Geometry check sheet. Reference: the model listing, model coordinates, mm. A direction names the side the tool comes from. Give positions to 0.01 mm unless a question says otherwise; leave off trailing zeros. Order: outer loops, then holes, each group sorted by start corner. A loop starts at its lowest first (then second) coordinate and runs counter-clockwise, first axis right, second up. Notation, with made-up numbers: M 55,17.25 L 68,17.25 A27 ccw 68,36.25 Z; hole C -36,-24.75 d5. An arc over 180 degrees is marked long. Answer as CSV lines item,"result". Start each with the question number.
Q1. Go/stop test with flat-tipped pins: pin 1 (6.5 mm diameter, centred on x = 4.5, y = 51.5, fed in from -Z); pin 2 (6 mm diameter, centred on x = -1.5, z = 31.5, fed in from +Y); pin 3 (5 mm diameter, centred on x = -20, z = 32, fed in from -Y). Record where each tip stops, or that it passes through.
Q2. Section check D-D, the plane y = 57. Record the boundary of the cut face in (x, z).
Q3. Section check A-A, the plane y = 43. Record the boundary of the cut face in (x, z) (3 decimals).
Q4. Thickness scan on line 1 (Y direction, x = -26, z = 23.5); line 2 (Y direction, x = -19.5, z = 15.5); line 3 (Y direction, x = 3, z = 13). Record the ranges inside material, lowest first.
Q5. Set-up check for faces 4 (the flat face through (4, 44.8, -2)), 5 (the flat face through (4, 15.2, -2)), 6 (the flat face through (-38, 41.8, 34)), 7 (the flat face through (-13, 30, 13.75)): record each of +Z, -Z, +X, -X, +Y, -Y from which the full face is reachable in a straight line by a thin tool's end or side.
Q6. Mould release check, pull along X, two halves, no side actions. Record for faces 1 (the flat face through (-10, 56, 28)), 2 (the cylindrical face through (2.54, 3.55, 24.71)), 3 (the flat face through (-19, -4, 16)): +X half, -X half, draft (parallel to the pull), parting line (faces both ways), or undercut.
Q7. Section check C-C, the plane x = -4. Record the boundary of the cut face in (y, z), then the cut area to 3 significant figures.
Q8. Section check B-B, the plane z = 18.5. Count the separate pieces of the cut face and the enclosed holes in it, then the cut area to 3 significant figures.
Autodesk Inventor part; units mm, degrees
ref_plane "YZ Plane" through (0, 0, 0) normal (1, 0, 0) x (0, 1, 0)
ref_plane "XZ Plane" through (0, 0, 0) normal (0, 1, 0) x (-1, 0, 0)
ref_plane "XY Plane" through (0, 0, 0) normal (0, 0, 1) x (1, 0, 0)
sketch "Эскиз1" plane through (0, 0, 0) normal (0, 1, 0) x (-1, 0, 0)
  line L0 (0, -4) -> (0, 0)
  line L1 (40, 31) -> (10, 31)
  line L2 (40, 31) -> (0, -4)
  line L3 (10, 31) -> (10, 8.75)
  line L4 (10, 8.75) -> (0, 0)
  dimension "d2" = 35
  dimension "d3" = 40
  dimension "d4" = 30
  dimension "d5" = 4
  dimension "d6" = 22.25
extrude "Выдавливание1" add sketch "Эскиз1" along normal blind 60
sketch "Эскиз2" plane through (-10, 0, 31) normal (1, 0, 0) x (0, 0, -1)
  line L0 (0, 0) -> (0, 60)
  line L1 (22.25, 0) -> (22.25, 60)
  line L2 (0, 53) -> (22.25, 53)
  line L3 (22.25, 53) -> (22.25, 7)
  line L4 (22.25, 7) -> (0, 7)
  line L5 (0, 7) -> (0, 53)
  point P0 (31, 0)
  point P1 (0, 30)
  dimension "d9" = 46
extrude "Выдавливание2" cut sketch "Эскиз2" against normal blind 2
sketch "Эскиз3" plane through (-12, 0, 31) normal (1, 0, 0) x (0, 0, -1)
  circle A0 centre (11.125, 43) radius 8.3
  circle A1 centre (11.125, 17) radius 8.3
  line L0 (11.125, 17) -> (11.125, 43) construction
  line L1 (0, 7) -> (0, 53)
  line L2 (0, 53) -> (22.25, 53)
  point P0 (31, 0)
  point P1 (11.125, 30)
  point P2 (0, 30)
  point P3 (11.125, 53)
  dimension "d12" = 16.6
  dimension "d13" = 26
extrude "Выдавливание3" cut sketch "Эскиз3" against normal through all
sketch "Эскиз4" plane through (-12, 0, 31) normal (1, 0, 0) x (0, 0, -1)
  line L0 (22.25, 53) -> (22.25, 7)
  line L1 (17.25, 36) -> (22.25, 36)
  line L2 (22.25, 36) -> (22.25, 24)
  line L3 (22.25, 24) -> (17.25, 24)
  line L4 (17.25, 24) -> (17.25, 36)
  line L5 (0, 36) -> (5, 36)
  line L6 (5, 36) -> (5, 24)
  line L7 (5, 24) -> (0, 24)
  line L8 (0, 24) -> (0, 36)
  line L9 (0, 7) -> (0, 53)
  point P0 (31, 0)
  point P1 (0, 30)
  dimension "d16" = 5
  dimension "d17" = 12
extrude "Выдавливание4" cut sketch "Эскиз4" against normal blind 1.4
sketch "Эскиз5" plane through (0, 0, 0) normal (1, 0, 0) x (0, 0, -1)
  line L0 (4, 0) -> (4, 60)
  line L1 (0, 44.8) -> (4, 44.8)
  line L2 (4, 44.8) -> (4, 15.2)
  line L3 (4, 15.2) -> (0, 15.2)
  line L4 (0, 15.2) -> (0, 44.8)
  line L5 (0, 0) -> (0, 60)
  point P0 (4, 30)
  dimension "d20" = 29.6
extrude "Выдавливание5" add sketch "Эскиз5" along normal blind 8
sketch "Эскиз6" plane through (-40, 0, 31) normal (0, 0, 1) x (1, 0, 0)
  line L0 (0, 0) -> (0, 60)
  line L1 (0, 15.2) -> (4, 15.2)
  line L2 (4, 15.2) -> (4, 41.8)
  line L3 (4, 41.8) -> (0, 41.8)
  line L4 (0, 41.8) -> (0, 15.2)
  point P0 (40, 0)
  point P1 (0, 30)
  dimension "d23" = 4
  dimension "d24" = 26.6
  dimension "d37" = 14.8
extrude "Выдавливание6" add sketch "Эскиз6" along normal blind 5
sketch "Эскиз7" plane through (0, 0, 0) normal (0, -1, 0) x (1, 0, 0)
  line L0 (-9.1664, 4.0206) -> (-6.5324, 7.0309)
  line L1 (-10, 8.75) -> (0, 0)
  line L2 (0, -4) -> (-40, 31)
  line L3 (-9.1664, 4.0206) -> (-30.8406, 22.9855)
  line L4 (-17.8, 11.575) -> (-36.7714, 28.175)
  line L5 (-30.8406, 22.9855) -> (-28.2066, 25.9958)
  line L6 (-28.2066, 25.9958) -> (-6.5324, 7.0309)
  dimension "d28" = 4
  dimension "d29" = 28.8
  dimension "d30" = 12.18
extrude "Выдавливание7" add sketch "Эскиз7" along normal blind 4
sketch "Эскиз8" plane through (0, 60, 0) normal (0, 1, 0) x (1, 0, 0)
  line L0 (-9.1664, -4.0206) -> (-6.5324, -7.0309)
  line L1 (-6.5324, -7.0309) -> (-28.2066, -25.9958)
  line L2 (-28.2066, -25.9958) -> (-30.8406, -22.9855)
  line L3 (-30.8406, -22.9855) -> (-9.1664, -4.0206)
  point P0 (0, 0)
extrude "Выдавливание8" add sketch "Эскиз8" along normal blind 4
sketch "Эскиз9" plane through (-40, 0, 31) normal (0, 0, 1) x (1, 0, 0)
  line L0 (0, 41.8) -> (4, 41.8)
  line L1 (4, 41.8) -> (4, 15.2)
  line L2 (4, 15.2) -> (0, 15.2)
  line L3 (0, 0) -> (0, 15.2)
  line L4 (0, 0) -> (30, 0)
  line L5 (30, 0) -> (30, 7)
  line L6 (30, 7) -> (28, 7)
  line L7 (28, 7) -> (28, 24)
  line L8 (28, 24) -> (26.6, 24)
  line L9 (26.6, 24) -> (26.6, 36)
  line L10 (26.6, 36) -> (28, 36)
  line L11 (28, 36) -> (28, 53)
  line L12 (28, 53) -> (30, 53)
  line L13 (30, 53) -> (30, 60)
  line L14 (0, 60) -> (30, 60)
  line L15 (0, 41.8) -> (0, 60)
  point P0 (40, 0)
extrude "Выдавливание9" add sketch "Эскиз9" along normal blind 1
sketch "Эскиз10" plane through (-13.4, 0, 31) normal (1, 0, 0) x (0, 0, -1)
  line L0 (5, 24) -> (-1, 24)
  line L1 (5, 36) -> (5, 24)
  line L2 (-1, 36) -> (5, 36)
  line L3 (-1, 24) -> (-1, 36)
  point P0 (31, 0)
extrude "Выдавливание10" cut sketch "Эскиз10" against normal blind 4
sketch "Эскиз12" plane through (0, 0, 0) normal (0, -1, 0) x (1, 0, 0)
  line L0 (-10, 8.75) -> (-10, 32)
  line L1 (0, 0) -> (8, 0)
  line L2 (-10, 8.75) -> (0, 0)
  line L3 (0, 0) -> (8, 0)
  line L4 (8, 0) -> (8, 8.75)
  line L5 (8, 8.75) -> (-10, 8.75)
extrude "Выдавливание11" add sketch "Эскиз12" against normal up to surface (60 mm away)
sketch "Эскиз13" plane through (0, 60, 0) normal (0, 1, 0) x (1, 0, 0)
  line L0 (-10, -32) -> (-10, -8.75)
  line L1 (-10, -8.75) -> (8, -8.75)
  line L2 (8, -8.75) -> (-10, -24.5)
  line L3 (-10, -8.75) -> (-12, -8.75)
  line L4 (-10, -8.75) -> (-10, -24.5)
  line L5 (0, 4) -> (-9.1664, -4.0206)
  point P0 (0, 0)
extrude "Выдавливание12" add sketch "Эскиз13" against normal up to surface (7 mm away)
sketch "Эскиз16" plane through (0, 0, 0) normal (0, -1, 0) x (1, 0, 0)
  line L0 (-10, 8.75) -> (-10, 32)
  line L1 (-10, 32) -> (8, 32)
  line L2 (8, 0) -> (8, 8.75)
  line L3 (8, 32) -> (8, 8.75)
  line L4 (-10, 8.75) -> (-12, 8.75)
  line L5 (8, 8.75) -> (-10, 8.75)
  line L6 (-10, 8.75) -> (-10, 32)
  point P0 (0, 0)
extrude "Выдавливание15" add sketch "Эскиз16" against normal blind 7
sketch "Эскиз17" plane through (8, 44.8, 0) normal (0, 0, -1) x (-1, 0, 0)
  line L0 (8, 15.2) -> (0, 15.2)
  line L1 (8, -44.8) -> (0, -44.8)
  point P0 (4, 6.2)
  point P1 (4, -35.8)
  point P2 (4, 15.2)
  dimension "d58" = 9
  dimension "d59" = 9
hole "Отверстие1" at (4, 51, 0) at (4, 9, 0) direction (0, 0, 1) diameter 2.8 end through all
sketch "Эскиз19" plane through (0, 0, 0) normal (0, -1, 0) x (1, 0, 0)
  line L0 (0, -4) -> (8, -4)
  line L1 (-40, 32) -> (-40, 36)
  line L2 (-40, 32) -> (8, 32)
  point P0 (0, 0)
  point P1 (-15, 24)
  point P2 (0, 6)
  point P3 (2, 26)
  dimension "d67" = 10
  dimension "d68" = 25
  dimension "d69" = 40
  dimension "d72" = 42
  dimension "d73" = 30
  dimension "d74" = 28
hole "Отверстие2" at (-15, 0, 24) at (0, 0, 6) at (2, 0, 26) direction (0, 1, 0) diameter 2.8 depth 7
properties part number "Sensor" material "Пластик АБС"
Answer block:
1,pin 1,"stops at z = 0"
1,pin 2,"stops at y = 7"
1,pin 3,"stops at y = 0"
2,outline,"M -40,31 L 0,-4 L 0,0 L 8,0 L 8,8.75 L -10,24.5 L -10,32 L -40,32 Z"
3,outline,"M -40,31 L -36.771,28.175 L -12,28.175 L -12,32 L -40,32 Z; M -17.8,11.575 L 0,-4 L 8,-4 L 8,8.75 L -12,8.75 L -12,11.575 Z"
4,line 1,"y = -4 to 9.53, 24.47 to 35.53, 50.47 to 64"
4,line 2,"y = -4 to 9.95, 24.05 to 35.95, 50.05 to 64"
4,line 3,"y = 0 to 7, 53 to 60"
5,face 4,"-Z, +X, +Y"
5,face 5,"-Z, +X, -Y"
5,face 6,"+Z, +X, -X, +Y"
5,face 7,"+X"
6,face 1,"+X half"
6,face 2,"undercut"
6,face 3,"draft"
7,outline,"M 0,-0.5 L 60,-0.5 L 60,19.25 L 53,19.25 L 53,8.75 L 7,8.75 L 7,32 L 0,32 Z"
7,area,"791 mm2"
8,separate pieces,"3"
8,enclosed holes,"0"
8,area,"624 mm2"
